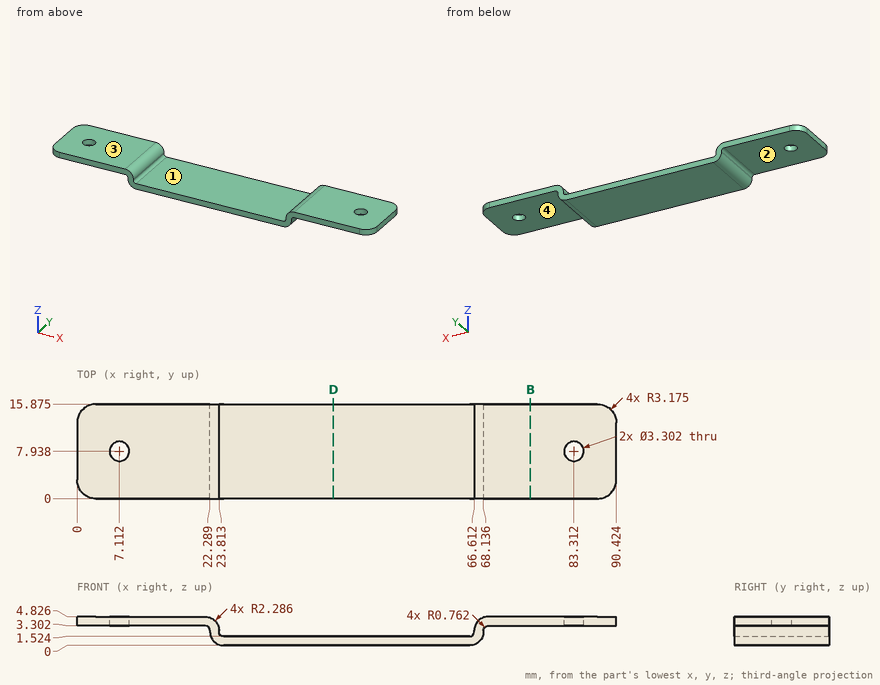
Job drawing, mm, ordinate dimensions from the low corner. One solid piece. A direction names the side the tool comes from. Give positions to 0.01 mm unless a question says otherwise; leave off trailing zeros. Order: outer loops, then holes, each group sorted by start corner. A loop starts at its lowest first (then second) coordinate and runs counter-clockwise, first axis right, second up. Notation, with made-up numbers: M 15.25,65.25 L 40.25,65.25 A36 ccw 40.25,103.25 Z; hole C -20,59 d8. An arc over 180 degrees is marked long. Return JSON: item names as keys, results as strings.
Q1. Band-saw the part on D-D (x = 43). Give the cut face in (y, z) (1 decimal).
Answer list:
{"outline": "M 0,0 L 15.9,0 L 15.9,1.5 L 0,1.5 Z"}
Q2. Wall check: probe 1 along X at (y, z) = (5.5, 2.7); probe 2 along Z at (x, y) = (20, 10) (1 decimal); probe 3 along X at (y, z) = (1.5, 2.2) (1 decimal). Give the ranges that are in metal, low to high. Write a range as from..to.
Answer list:
{"probe 1": "x = 22.27..23.81, 66.62..68.15", "probe 2": "z = 3.3..4.8", "probe 3": "x = 22.3..23.8, 66.6..68.1"}
Q3. Flat gauge pins, fed straight in: pin 1 (1 mm diameter, centred on y = 14, z = 3, fed in from -X); pin 2 (2 mm diameter, centred on x = 83.31, y = 7.94, fed in from -Z); pin 3 (1 mm diameter, centred on x = 77.5, y = 12, fed in from -Z). Where does each tip first touch, or does it go through?
Answer list:
{"pin 1": "stops at x = 0.13", "pin 2": "passes through", "pin 3": "stops at z = 3.3"}
Q4. 3-axis set-ups, long thin cutter, end or side, ignore diameter. For the marked faces 1, 2, 3 and 4: which of +Z, -Z, +X, -X, +Y, -Y reach the whole face in a straight line?
Answer list:
{"face 1": "+Z, +Y, -Y", "face 2": "-Z, -X, +Y, -Y", "face 3": "+Z, +X, -X, +Y, -Y", "face 4": "-Z, +X, +Y, -Y"}
Q5. Band-saw the part on B-B (x = 76). Give the cut face in (y, z) (1 decimal), then the cut area to 3 significant figures.
Answer list:
{"outline": "M 0,3.3 L 15.9,3.3 L 15.9,4.8 L 0,4.8 Z", "area": "24.2 mm^2"}
